Check sheet for the modelled part. Datum: model origin and axes. Units: mm. A direction names the side the tool comes from. Give positions to 0.01 mm unless a question says otherwise; leave off trailing zeros. Loops run counter-clockwise (first coordinate to the right, second up) from the corner with the lowest first, then second, coordinate; pieces in that order, holes last. Notation, with made-up numbers: M 83,3.5 L 87,3.5 A19 ccw 87,29.5 Z; hole C 68.5,7.5 d6. An arc over 180 degrees is marked long. Use one line per item in the form item = value.
from build123d import *

# Parameters (mm, degrees)
EXTRUDE_1_DEPTH = 5
SKETCH_3_W      = 70
SKETCH_3_H      = 10
SKETCH_3_R      = 2.5
EXTRUDE_2_DEPTH = 5
EXTRUDE_START   = -5
SKETCH_4_W      = 12.5
SKETCH_4_H      = 10
SKETCH_4_R      = 2.5
EXTRUDE_3_DEPTH = 5


with BuildPart() as part:
    # 草图1 → 凸台-拉伸1 (new, symmetric)
    with BuildSketch(Plane.XY):
        with BuildLine():
            Line((16.45, 0), (22.5, 0))
            Line((22.5, 0), (22.5, -30))
            Line((22.5, -30), (-22.5, -30))
            Line((-22.5, -30), (-22.5, 0))
            Line((-22.5, 0), (-16.45, 0))
            ThreePointArc((-16.45, 0), (0, -16.45), (16.45, 0))
        make_face()
    extrude(amount=EXTRUDE_1_DEPTH, both=True)

    # 草图3 → 凸台-拉伸2 (add)
    with BuildSketch(Plane.XZ.offset(30)):
        Rectangle(SKETCH_3_W, SKETCH_3_H)
        with Locations((-30, 0)):
            Circle(SKETCH_3_R, mode=Mode.SUBTRACT)
        with Locations(Location((30, 0, 0), (0, 0, 180))):
            Circle(SKETCH_3_R, mode=Mode.SUBTRACT)
    extrude(amount=-EXTRUDE_2_DEPTH)

    # 草图4 → 凸台-拉伸3 (add)
    # profile 1 of 2: a face of its own
    with BuildSketch(Plane(origin=(0, 0, 0), x_dir=(1, 0, 0), z_dir=(0, 1, 0)).offset(EXTRUDE_START)):
        with Locations((-28.75, 0)):
            Rectangle(SKETCH_4_W, SKETCH_4_H)
        with Locations((-30, 0)):
            Circle(SKETCH_4_R, mode=Mode.SUBTRACT)
    # profile 2 of 2: a face of its own
    with BuildSketch(Plane(origin=(0, 0, 0), x_dir=(1, 0, 0), z_dir=(0, 1, 0)).offset(EXTRUDE_START)):
        with Locations((28.75, 0)):
            Rectangle(SKETCH_4_W, SKETCH_4_H)
        with Locations(Location((30, 0, 0), (0, 0, 180))):
            Circle(SKETCH_4_R, mode=Mode.SUBTRACT)
    extrude(amount=EXTRUDE_3_DEPTH)


solid = part.part
1) Set-up check for faces 1 (the face through (32.5, -27.5, -0.1)), 2 (the face through (-27, -25, 0)), 3 (the face through (27, -5, 0)): record each of +Z, -Z, +X, -X, +Y, -Y from which the full face is reachable in a straight line by a thin tool's end or side.
Evaluation:
face_1 = +Y, -Y
face_2 = +Z, -Z, -X
face_3 = +Z, -Z, +X
2) Section check A-A (z = 0). State how many separate pieces and enclosed holes the cut face has, then the cut area to 3 significant figures.
Evaluation:
separate_pieces = 5
enclosed_holes = 0
area = 1,070 mm^2
3) Scan lines: line 1 (Z direction, x = -30, y = -2.85); line 2 (Y direction, x = -30.5, z = 3); line 3 (X direction, y = -2.5, z = 1.5). Record each from-to range of solid material in increasing order.
Evaluation:
line_1 = -5 to -2.5, 2.5 to 5
line_2 = -30 to -25, -5 to 0
line_3 = -35 to -32, -28 to -16.26, 16.26 to 28, 32 to 35
4) Section check B-B (x = 30). Record the cut outline in (y, z), then the cut area to 3 significant figures.
Evaluation:
outline = M -30,-5 L -25,-5 L -25,-2.5 L -30,-2.5 Z; M -30,2.5 L -25,2.5 L -25,5 L -30,5 Z; M -5,-5 L 0,-5 L 0,-2.5 L -5,-2.5 Z; M -5,2.5 L 0,2.5 L 0,5 L -5,5 Z
area = 50.0 mm^2
5) Section check C-C (y = -26.5). Record the cut outline in (x, z).
Evaluation:
outline = M -35,-5 L 35,-5 L 35,5 L -35,5 Z; hole C -30,0 d5; hole C 30,0 d5
6) Section check D-D (y = -11.5). Record the cut outline in (x, z), then the cut area to 3 significant figures.
Evaluation:
outline = M -22.5,-5 L -11.76,-5 L -11.76,5 L -22.5,5 Z; M 11.76,-5 L 22.5,-5 L 22.5,5 L 11.76,5 Z
area = 215 mm^2
7) Release check for a two-part mould opening along Y. For faces 4 (the face through (-22.5, -15, 0)), 5 (the face through (-32.5, -27.5, 0.1)), 6 (the face through (-0.362, -16.446, 0.07)) record: pulls with the +Y half, pulls with the -Y half, needs draft (parallel to the pull), parting line crosses it, or undercut.
Evaluation:
face_4 = undercut
face_5 = needs draft
face_6 = pulls with the +Y half
8) Depth check by flat-ended pin: pin 1 Ø6 at (x, z) = (30, 0) entering from -Y; pin 2 Ø1.5 at (y, z) = (-17, 3.5) entering from -X; pin 3 Ø1 at (y, z) = (-11, -1.5) entering from +X; pin 4 Ø4.5 at (x, z) = (-30, 0) entering from -Y. Enter the tip coordinate at first touch or a pass-through.
Evaluation:
pin_1 = -30
pin_2 = -22.5
pin_3 = 22.5
pin_4 = through
